```python
from build123d import *

# Parameters (mm, degrees)
SKETCH1_W           = 70
SKETCH1_H           = 30
BOSS_EXTRUDE1_DEPTH = 20
SKETCH8_W           = 20
SKETCH8_H           = 20
SKETCH8_R           = 2.75
BOSS_EXTRUDE5_DEPTH = 5
FILLET3_R           = 5
SKETCH9_W           = 35
SKETCH9_H           = 40
CUT_EXTRUDE5_DEPTH  = 5


with BuildPart() as part:
    # Sketch1 → Boss-Extrude1 (new body)
    with BuildSketch(Plane(origin=(0, 0, 0), x_dir=(1, 0, 0), z_dir=(0, 1, 0))):
        with Locations((35, 15)):
            Rectangle(SKETCH1_W, SKETCH1_H)
    extrude(amount=BOSS_EXTRUDE1_DEPTH)

    # Sketch8 → Boss-Extrude5 (add)
    with BuildSketch(Plane(origin=(70, 0, 0), x_dir=(0, 0, -1), z_dir=(1, 0, 0))):
        with Locations((-10, 10)):
            Rectangle(SKETCH8_W, SKETCH8_H)
        with Locations((-10, 10)):
            Circle(SKETCH8_R, mode=Mode.SUBTRACT)
    boss_extrude5 = extrude(amount=-BOSS_EXTRUDE5_DEPTH)

    # Mirror1: Boss-Extrude5 across plane
    add(boss_extrude5.mirror(Plane.XY.offset(-15)))

    # Fillet3
    fillet3_edges = [part.edges().sort_by_distance(p)[0] for p in [
        (65, 10, 0),
        (65, 10, -30),
        (0, 0, -15),
    ]]
    fillet(fillet3_edges, radius=FILLET3_R)

    # Sketch9 → Cut-Extrude5 (cut)
    with BuildSketch(Plane(origin=(0, 20, 0), x_dir=(1, 0, 0), z_dir=(0, 1, 0))):
        with Locations((47.5, 15)):
            Rectangle(SKETCH9_W, SKETCH9_H)
    extrude(amount=-CUT_EXTRUDE5_DEPTH, mode=Mode.SUBTRACT)


solid = part.part
```
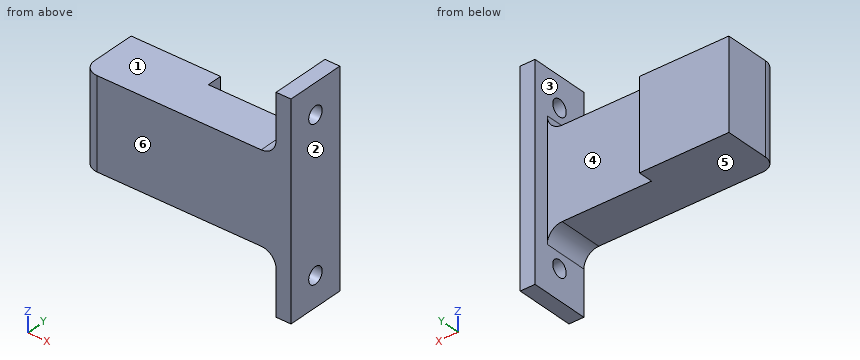
Model file for the job. Use its own axes, mm. Face numbers are marked on the shaded views. A direction names the side the tool comes from. Give positions to 0.01 mm unless a question says otherwise; leave off trailing zeros. Write each loop counter-clockwise with the first axis right and the second up, starting at its lowest first coordinate (ties: lowest second). Pieces come first, ordered by that corner, then holes. Notation, with made-up numbers: M -39.75,-28 L -27.75,-28 A10 ccw -27.75,-16 Z; hole C 88.25,72.25 d11. An arc over 180 degrees is marked long. Use a Markdown table: item, result.
1) Pull direction X, two halves, no side cores. Call the marked faces 1, 2 and 3: +X half, -X half, draft (parallel to the pull), parting line (faces both ways), or undercut.
Responses:
| item | result |
|---|---|
| face 1 | draft |
| face 2 | +X half |
| face 3 | undercut |
2) Pin check, flat tips, straight feed: pin 1 (6 mm diameter, centred on x = 22, y = 5, fed in from +Z); pin 2 (10.5 mm diameter, centred on x = 52.5, z = -5.5, fed in from +Y); pin 3 (6 mm diameter, centred on x = 30.5, y = 12, fed in from -Z). Stop position of each tip, or through.
Responses:
| item | result |
|---|---|
| pin 1 | stops at z = 0 |
| pin 2 | stops at y = 15 |
| pin 3 | stops at z = -30 |
3) Drill centre lines: line 1 (Y direction, x = 68.3, z = 10); line 2 (X direction, y = 17.5, z = -46); line 3 (Z direction, x = 50.5, y = 10.5). Where is each one in solid material? Low to high. Write a range as from..to.
Responses:
| item | result |
|---|---|
| line 1 | y = 0..7.25, 12.75..20 |
| line 2 | x = 65..70 |
| line 3 | z = -30..0 |
4) Cut at C-C (z = -2). List the corners of the cut face in (x, y), and give its area (3 significant figures).
Responses:
| item | result |
|---|---|
| outline | M 0,5 A5 ccw 5,0 L 70,0 L 70,20 L 65,20 L 65,15 L 30,15 L 30,20 L 0,20 Z |
| area | 1,220 mm2 |
5) Tool access for the marked faces 4, 5 and 6: list every direction of +Z, -Z, +X, -X, +Y, -Y with a clear straight run to the whole face (end or side of a thin tool).
Responses:
| item | result |
|---|---|
| face 4 | +Z, -Z, +Y |
| face 5 | -Z, -X, +Y, -Y |
| face 6 | +Z, -Z, +X, -X, -Y |
6) Cut at D-D (x = 17.5). List the corners of the cut face in (y, z).
Responses:
| item | result |
|---|---|
| outline | M 0,-30 L 20,-30 L 20,0 L 0,0 Z |
7) Cut at A-A (z = -40). List the corners of the cut face in (x, y), and give its area (3 significant figures).
Responses:
| item | result |
|---|---|
| outline | M 65,0 L 70,0 L 70,7.25 L 65,7.25 Z; M 65,12.75 L 70,12.75 L 70,20 L 65,20 Z |
| area | 72.5 mm2 |
8) Cut at B-B (y = 10). List the corners of the cut face in (x, z), and give its area (3 significant figures).
Responses:
| item | result |
|---|---|
| outline | M 0,-30 L 60,-30 A5 cw 65,-35 L 65,-37.25 L 70,-37.25 L 70,7.25 L 65,7.25 L 65,5 A5 cw 60,0 L 0,0 Z; M 65,-50 L 70,-50 L 70,-42.75 L 65,-42.75 Z; M 65,12.75 L 70,12.75 L 70,20 L 65,20 Z |
| area | 2,260 mm2 |
